Autodesk Inventor part; units mm, degrees
ref_plane "YZ Plane" through (0, 0, 0) normal (1, 0, 0) x (0, 1, 0)
ref_plane "XZ Plane" through (0, 0, 0) normal (0, 1, 0) x (-1, 0, 0)
ref_plane "XY Plane" through (0, 0, 0) normal (0, 0, 1) x (1, 0, 0)
sketch "Sketch1" plane through (0, 0, 0) normal (1, 0, 0) x (0, 1, 0)
  line L0 (42, 70) -> (-42, 70)
  line L1 (-42, 70) -> (-42, -70)
  line L2 (-42, -70) -> (42, -70)
  line L3 (42, -70) -> (42, 70)
  line L4 (0, 70) -> (0, -70) construction
  line L5 (-42, 0) -> (42, 0) construction
  circle A0 centre (-37, 65) radius 1.75
  circle A1 centre (-37, -65) radius 1.75
  circle A2 centre (33, 65) radius 1.75
  circle A3 centre (-37, -65) radius 1.75
  circle A4 centre (33, -65) radius 1.75
  point P0 (0, 0)
  point P1 (0, 0)
  dimension "d0" = 84
  dimension "d1" = 140
  dimension "d2" = 3.5
  dimension "d3" = 5
  dimension "d4" = 5
  dimension "d5" = 3.5
  dimension "d6" = 9
  dimension "d7" = 5
extrude "Extrusion1" add sketch "Sketch1" along normal blind 4
sketch "Sketch2" plane through (4, 0, 0) normal (1, 0, 0) x (0, 0, -1)
  line L0 (-34, 4) -> (34, 4) construction
  line L1 (34, 4) -> (34, -28) construction
  line L2 (34, -28) -> (-34, -28) construction
  line L3 (-34, -28) -> (-34, 4) construction
  line L4 (-70, 42) -> (-70, -42) construction
  line L5 (70, 42) -> (-70, 42) construction
  line L6 (0, 42) -> (0, -42) construction
  line L7 (-70, -42) -> (70, -42) construction
  circle A0 centre (-34, -28) radius 1.5
  circle A1 centre (-34, 4) radius 1.5
  circle A2 centre (34, 4) radius 1.5
  circle A3 centre (34, -28) radius 1.5
  point P0 (0, 0)
  dimension "d10" = 36
  dimension "d11" = 32
  dimension "d12" = 14
  dimension "d13" = 3
  dimension "d14" = 3
  dimension "d15" = 3
  dimension "d16" = 3
extrude "Extrusion2" cut sketch "Sketch2" against normal blind 4
properties part number "electronics_case_panel"
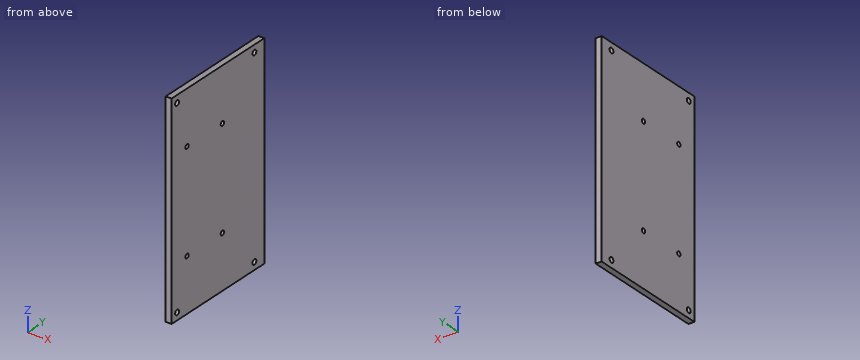
Source: CAD feature listing. Evaluate the final solid. Frame: model axes, mm. Coordinates: 2 decimals unless noted, no trailing zeros. Loops run counter-clockwise (first coordinate to the right, second up) from the corner with the lowest first, then second, coordinate; pieces in that order, holes last. Notation, with made-up numbers: (57.5, -31) -> (81.5, -31) arc R11 ccw to (81.5, -21) -> close; hole circle Ø2 at (54, 76). An arc over 180 degrees is marked (long way). Answer in a Markdown table with one row per item. Add a question column.
Q1. Ray query, line 1 along Y through (x, z) = (1.3, 65); line 2 along Y through (x, z) = (1.35, -34); line 3 along Z through (x, y) = (1.75, -37). Return the intervals inside material, ascending.
Q2. Section A-A on z = -34. Return the cut outline in (x, y).
Q3. Section B-B on y = 4. Return the cut outline in (x, z), and give its area (3 significant figures).
Q4. Contact query for a flat-ended pin moving along its axis: pin 1 Ø2.5 at (y, z) = (4, -34) entering from +X. Output: stop coordinate, or through.
Computed values:
| question | item | result |
|---|---|---|
| 1 | line 1 | y = -42 to -38.75, -35.25 to 31.25, 34.75 to 42 |
| 1 | line 2 | y = -42 to -29.5, -26.5 to 2.5, 5.5 to 42 |
| 1 | line 3 | z = -70 to -66.75, -63.25 to 63.25, 66.75 to 70 |
| 2 | outline | (0, -42) -> (4, -42) -> (4, -29.5) -> (0, -29.5) -> close; (0, -26.5) -> (4, -26.5) -> (4, 2.5) -> (0, 2.5) -> close; (0, 5.5) -> (4, 5.5) -> (4, 42) -> (0, 42) -> close |
| 3 | outline | (0, -70) -> (4, -70) -> (4, -35.5) -> (0, -35.5) -> close; (0, -32.5) -> (4, -32.5) -> (4, 32.5) -> (0, 32.5) -> close; (0, 35.5) -> (4, 35.5) -> (4, 70) -> (0, 70) -> close |
| 3 | area | 536 mm^2 |
| 4 | pin 1 | passes through |
